```python
from build123d import *

# Parameters (mm, degrees)
SKETCH16_R           = 2.5
F_20X40XR1_5_2_DEPTH = 300


with BuildPart() as part:
    # Sketch16 → 铝型材 20X40XR1.5(2) (new body)
    with BuildSketch(Plane(origin=(-53.342500755, -1.452155193, 0), x_dir=(0, 1, 0), z_dir=(1, 0, 0))):
        with BuildLine():
            Line((-3.6, 10), (-3.6, 9.5))
            Line((-3.6, 9.5), (-3.1, 9.5))
            Line((-3.1, 9.5), (-3.1, 8.5))
            Line((-3.1, 8.5), (-5.5, 8.5))
            Line((-5.5, 8.5), (-5.5, 6.65))
            Line((-5.5, 6.65), (-2.75, 3.9))
            Line((-2.75, 3.9), (2.75, 3.9))
            Line((2.75, 3.9), (5.5, 6.65))
            Line((5.5, 6.65), (5.5, 8.5))
            Line((5.5, 8.5), (3.1, 8.5))
            Line((3.1, 8.5), (3.1, 9.5))
            Line((3.1, 9.5), (3.6, 9.5))
            Line((3.6, 9.5), (3.6, 10))
            Line((3.6, 10), (8.5, 10))
            ThreePointArc((8.5, 10), (9.560660172, 9.560660172), (10, 8.5))
            Line((10, 8.5), (10, 3.6))
            Line((10, 3.6), (9.5, 3.6))
            Line((9.5, 3.6), (9.5, 3.1))
            Line((9.5, 3.1), (8.5, 3.1))
            Line((8.5, 3.1), (8.5, 5.5))
            Line((8.5, 5.5), (6.65, 5.5))
            Line((6.65, 5.5), (3.9, 2.75))
            Line((3.9, 2.75), (3.9, -2.75))
            Line((3.9, -2.75), (6.65, -5.5))
            Line((6.65, -5.5), (8.5, -5.5))
            Line((8.5, -5.5), (8.5, -3.1))
            Line((8.5, -3.1), (9.5, -3.1))
            Line((9.5, -3.1), (9.5, -3.6))
            Line((9.5, -3.6), (10, -3.6))
            Line((10, -3.6), (10, -16.4))
            Line((10, -16.4), (9.5, -16.4))
            Line((9.5, -16.4), (9.5, -16.9))
            Line((9.5, -16.9), (8.5, -16.9))
            Line((8.5, -16.9), (8.5, -14.5))
            Line((8.5, -14.5), (6.65, -14.5))
            Line((6.65, -14.5), (3.9, -17.25))
            Line((3.9, -17.25), (3.9, -22.75))
            Line((3.9, -22.75), (6.65, -25.5))
            Line((6.65, -25.5), (8.5, -25.5))
            Line((8.5, -25.5), (8.5, -23.1))
            Line((8.5, -23.1), (9.5, -23.1))
            Line((9.5, -23.1), (9.5, -23.6))
            Line((9.5, -23.6), (10, -23.6))
            Line((10, -23.6), (10, -28.5))
            ThreePointArc((10, -28.5), (9.560660172, -29.560660172), (8.5, -30))
            Line((8.5, -30), (3.6, -30))
            Line((3.6, -30), (3.6, -29.5))
            Line((3.6, -29.5), (3.1, -29.5))
            Line((3.1, -29.5), (3.1, -28.5))
            Line((3.1, -28.5), (5.5, -28.5))
            Line((5.5, -28.5), (5.5, -26.65))
            Line((5.5, -26.65), (2.75, -23.9))
            Line((2.75, -23.9), (-2.75, -23.9))
            Line((-2.75, -23.9), (-5.5, -26.65))
            Line((-5.5, -26.65), (-5.5, -28.5))
            Line((-5.5, -28.5), (-3.1, -28.5))
            Line((-3.1, -28.5), (-3.1, -29.5))
            Line((-3.1, -29.5), (-3.6, -29.5))
            Line((-3.6, -29.5), (-3.6, -30))
            Line((-3.6, -30), (-8.5, -30))
            ThreePointArc((-8.5, -30), (-9.560660172, -29.560660172), (-10, -28.5))
            Line((-10, -28.5), (-10, -23.6))
            Line((-10, -23.6), (-9.5, -23.6))
            Line((-9.5, -23.6), (-9.5, -23.1))
            Line((-9.5, -23.1), (-8.5, -23.1))
            Line((-8.5, -23.1), (-8.5, -25.5))
            Line((-8.5, -25.5), (-6.65, -25.5))
            Line((-6.65, -25.5), (-3.9, -22.75))
            Line((-3.9, -22.75), (-3.9, -17.25))
            Line((-3.9, -17.25), (-6.65, -14.5))
            Line((-6.65, -14.5), (-8.5, -14.5))
            Line((-8.5, -14.5), (-8.5, -16.9))
            Line((-8.5, -16.9), (-9.5, -16.9))
            Line((-9.5, -16.9), (-9.5, -16.4))
            Line((-9.5, -16.4), (-10, -16.4))
            Line((-10, -16.4), (-10, -3.6))
            Line((-10, -3.6), (-9.5, -3.6))
            Line((-9.5, -3.6), (-9.5, -3.1))
            Line((-9.5, -3.1), (-8.5, -3.1))
            Line((-8.5, -3.1), (-8.5, -5.5))
            Line((-8.5, -5.5), (-6.65, -5.5))
            Line((-6.65, -5.5), (-3.9, -2.75))
            Line((-3.9, -2.75), (-3.9, 2.75))
            Line((-3.9, 2.75), (-6.65, 5.5))
            Line((-6.65, 5.5), (-8.5, 5.5))
            Line((-8.5, 5.5), (-8.5, 3.1))
            Line((-8.5, 3.1), (-9.5, 3.1))
            Line((-9.5, 3.1), (-9.5, 3.6))
            Line((-9.5, 3.6), (-10, 3.6))
            Line((-10, 3.6), (-10, 8.5))
            ThreePointArc((-10, 8.5), (-9.560660172, 9.560660172), (-8.5, 10))
            Line((-8.5, 10), (-3.6, 10))
        make_face()
        Circle(SKETCH16_R, mode=Mode.SUBTRACT)
        with Locations((0, -20)):
            Circle(SKETCH16_R, mode=Mode.SUBTRACT)
        Polygon((8.85, -10), (2.75, -3.9), (-2.75, -3.9), (-8.85, -10), (-2.75, -16.1), (2.75, -16.1), align=None, mode=Mode.SUBTRACT)
    extrude(amount=F_20X40XR1_5_2_DEPTH)


solid = part.part
```
Geometry: final body of the model. Coordinates: model frame, mm. A direction names the side the tool comes from. Round coordinates to 2 decimals unless told otherwise and drop trailing zeros. Order: outer loops, then holes, each group sorted by start corner. A loop starts at its lowest first (then second) coordinate and runs counter-clockwise, first axis right, second up. Notation, with made-up numbers: (84.5, 27) -> (127.5, 27) arc R26 cw to (127.5, 61) -> close; hole circle Ø2 at (1, 8). An arc over 180 degrees is marked (long way). Use CSV: the item, a comma, the result in double quotes. Start each with the question number.
1) Material intervals for line 1 along Z through (x, y) = (146, -1); line 2 along Y through (x, z) = (170, 8); line 3 along Z through (x, y) = (67, -8.75), sorted ascending. Write a range as from..to.
2) First-contact query: pin 1 Ø1 at (x, z) = (36, -22.5) entering from -Y; pin 2 Ø4.5 at (x, y) = (136, -1) entering from +Z; pin 3 Ø1.5 at (x, y) = (111, 1) entering from -Z; pin 4 Ø4 at (y, z) = (-1.45, 0) entering from -X. Flat tips, straight axial feed; report the tip coordinate or a pass-through.
3) Section B-B (x = 57). State how many separate pieces and enclosed holes the cut face has, and give its area (3 significant figures).
4) Set-up query: faces 4 (the face through (95, -1, -3.9)), 5 (the face through (95, 2.448, -20)), 6 (the face through (95, -5.352, 0)), 7 (the face through (246.657, 3, -5)), 8 (the face through (95, 8.548, -26)). Return all of +Z, -Z, +X, -X, +Y, -Y with unobstructed straight access to the full face (end or side cutting, diameter ignored); none if empty.
5) Section A-A (z = 0). Return the cut outline in (x, y).
6) Draft query along Y for faces 1 (the face through (95, -11.452, -10)), 2 (the face through (95, -1, -23.9)), 3 (the face through (95, 8.548, -10)). Return one class per face: +Y half, -Y half, draft (parallel to the pull), parting line (faces both ways), or undercut.
Returned:
1,line 1,"z = -23.9..-22.46, -17.54..-16.1, -3.9..-2.46, 2.46..3.9"
1,line 2,"y = -11.45..-6.95, 4.05..8.55"
1,line 3,"z = -30..-25.5, -14.5..-11.55, -8.45..-5.5, 5.5..10"
2,pin 1,"stops at y = -5.6"
2,pin 2,"stops at z = 3.9"
2,pin 3,"stops at z = -29.5"
2,pin 4,"passes through"
3,separate pieces,"1"
3,enclosed holes,"3"
3,area,"300 mm²"
4,face 4,"+X, -X"
4,face 5,"+X, -X, +Y"
4,face 6,"+X, -X, -Y"
4,face 7,"+Z, -Z, +X, +Y, -Y"
4,face 8,"+Z, -Z, +X, -X, +Y"
5,outline,"(-53.34, -5.35) -> (246.66, -5.35) -> (246.66, -3.95) -> (-53.34, -3.95) -> close; (-53.34, 1.05) -> (246.66, 1.05) -> (246.66, 2.45) -> (-53.34, 2.45) -> close"
6,face 1,"-Y half"
6,face 2,"undercut"
6,face 3,"+Y half"
